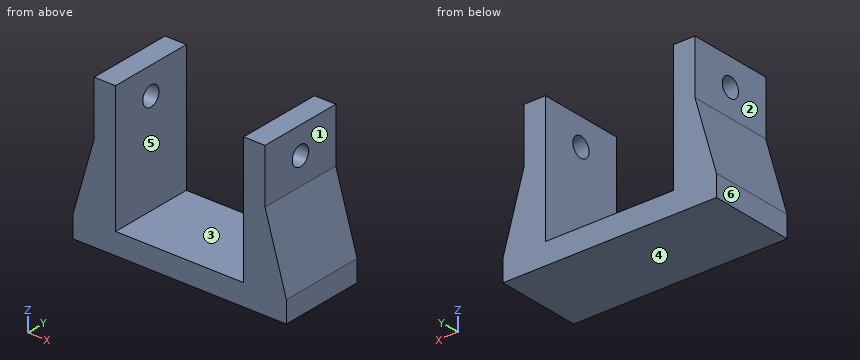
from build123d import *

# Parameters (mm, degrees)
F0_W     = 50
F0_H     = 20
F1_DEPTH = 5
F2_W     = 10
F2_H     = 20
F3_DEPTH = 30
F5_DEPTH = 20.001
F6_R     = 2.286
F7_DEPTH = 45.001


with BuildPart() as f1:
    # F0 (on Top) → F1 (new body)
    with BuildSketch(Plane.XY):
        Rectangle(F0_W, F0_H)
    extrude(amount=F1_DEPTH)

    # F2 (on face) → F3 (join)
    with BuildSketch(Plane.XY.offset(5)):
        with Locations((20, 0)):
            Rectangle(F2_W, F2_H)
        with Locations((-20, 0)):
            Rectangle(F2_W, F2_H)
    extrude(amount=F3_DEPTH)

    # F4 (on face) → F5 (cut, through all)
    with BuildSketch(Plane(origin=(0, 10, 0), x_dir=(-1, 0, 0), z_dir=(0, 1, 0))):
        Polygon((-25, 5), (-20, 22.3), (-20, 35), (-25, 35), align=None)
        Polygon((20, 35), (20, 22.3), (25, 5), (25, 35), align=None)
    extrude(amount=-F5_DEPTH, mode=Mode.SUBTRACT)

    # F6 (on face) → F7 (cut, through all)
    with BuildSketch(Plane(origin=(-20, 0, 0), x_dir=(0, -1, 0), z_dir=(-1, 0, 0))):
        with Locations((0, 28.65)):
            Circle(F6_R)
    extrude(amount=-F7_DEPTH, mode=Mode.SUBTRACT)


solid = f1.part
Work out the finished part from the listing and answer in its coordinate system (mm). Face numbers are marked on the shaded views. A direction names the side the tool comes from. Round coordinates to 2 decimals unless told otherwise and drop trailing zeros. Write each loop counter-clockwise with the first axis right and the second up, starting at its lowest first coordinate (ties: lowest second). Pieces come first, ordered by that corner, then holes. Notation, with made-up numbers: (17.5, 14.25) - (34.5, 14.25) arc R15 cw to (34.5, 21.25) - close; hole circle Ø4 at (63, 51.25). An arc over 180 degrees is marked (long way). Answer in a Markdown table with one row per item. Add a question column.
1. Given pin 1 (2 mm diameter, centred on y = 4.5, z = 15.5, fed in from -X); pin 2 (1 mm diameter, centred on y = -4, z = 27.5, fed in from -X); pin 3 (4 mm diameter, centred on x = 2.5, y = -0.5, fed in from +Z), each flat-ended and moving along its own axis, determine where each tip first touches the part or whether it passes through.
2. A cutting plane is placed at B-B, the plane z = 28.65. Determine the outline of the cut face in (x, y), and give its area (3 significant figures).
3. A cutting plane is placed at C-C, the plane x = -17.5. Determine the outline of the cut face in (y, z), and give its area (3 significant figures).
4. A cutting plane is placed at D-D, the plane z = 24.5. Determine the outline of the cut face in (x, y), and give its area (3 significant figures).
5. A cutting plane is placed at A-A, the plane y = 0. Determine the outline of the cut face in (x, z).
6. Find the intervals of material crossed by line 1 along Z through (x, y) = (-18.7, 0); line 2 along X through (y, z) = (2.5, 25.5); line 3 along Z through (x, y) = (1, -8), in increasing order. Write a range as from..to.
7. For the marked faces 1, 2 and 3, determine the directions among +Z, -Z, +X, -X, +Y, -Y from which every point of the face is accessible in a straight line to the end or side of a thin tool.
8. The mould has two halves that part along X. Classify the marked faces 4, 5 and 6: +X half, -X half, draft (parallel to the pull), parting line (faces both ways), or undercut.
Worked out:
| question | item | result |
|---|---|---|
| 1 | pin 1 | x = -22.25 |
| 1 | pin 2 | x = -20 |
| 1 | pin 3 | z = 5 |
| 2 | outline | (-20, -10) - (-15, -10) - (-15, -2.29) - (-20, -2.29) - close; (-20, 2.29) - (-15, 2.29) - (-15, 10) - (-20, 10) - close; (15, -10) - (20, -10) - (20, -2.29) - (15, -2.29) - close; (15, 2.29) - (20, 2.29) - (20, 10) - (15, 10) - close |
| 2 | area | 154 mm^2 |
| 3 | outline | (-10, 0) - (10, 0) - (10, 35) - (-10, 35) - close; hole circle Ø4.57 at (0, 28.65) |
| 3 | area | 684 mm^2 |
| 4 | outline | (-20, -10) - (-15, -10) - (-15, 10) - (-20, 10) - close; (15, -10) - (20, -10) - (20, 10) - (15, 10) - close |
| 4 | area | 200 mm^2 |
| 5 | outline | (-25, 0) - (25, 0) - (25, 5) - (20, 22.3) - (20, 26.36) - (15, 26.36) - (15, 5) - (-15, 5) - (-15, 26.36) - (-20, 26.36) - (-20, 22.3) - (-25, 5) - close; (-20, 30.94) - (-15, 30.94) - (-15, 35) - (-20, 35) - close; (15, 30.94) - (20, 30.94) - (20, 35) - (15, 35) - close |
| 6 | line 1 | 0..26.36, 30.94..35 |
| 6 | line 2 | -20..-15, 15..20 |
| 6 | line 3 | 0..5 |
| 7 | face 1 | +Z, +X, +Y, -Y |
| 7 | face 2 | +Z, -X, +Y, -Y |
| 7 | face 3 | +Z, +Y, -Y |
| 8 | face 4 | draft |
| 8 | face 5 | undercut |
| 8 | face 6 | -X half |
